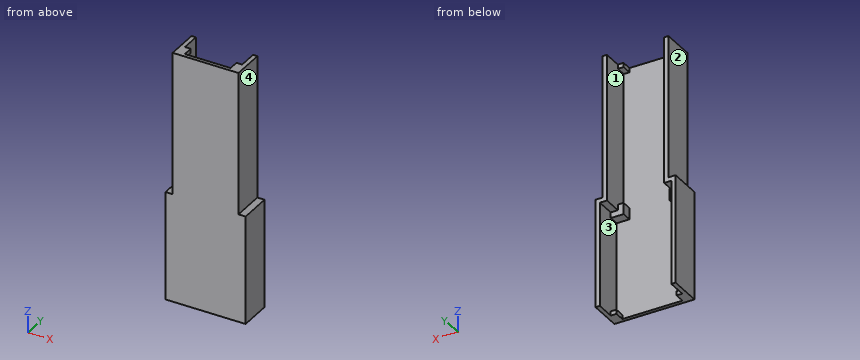
```python
from build123d import *

# Parameters (mm, degrees)
SKETCH1_W           = 46
SKETCH1_H           = 103
SKETCH1_W_2         = 56
SKETCH1_H_2         = 73
BOSS_EXTRUDE2_DEPTH = 2.5
BOSS_EXTRUDE3_DEPTH = 20
SKETCH4_W           = 3
SKETCH4_H           = 22.5
BOSS_EXTRUDE4_DEPTH = 5
SKETCH7_W           = 3
SKETCH7_H           = 22.5
BOSS_EXTRUDE5_DEPTH = 5
SKETCH8_W           = 4
SKETCH8_H           = 3
CUT_EXTRUDE1_DEPTH  = 13
SKETCH9_W           = 42
SKETCH9_H           = 3
CUT_EXTRUDE2_DEPTH  = 20
SKETCH10_W          = 32
SKETCH10_H          = 3
CUT_EXTRUDE3_DEPTH  = 20
SKETCH11_W          = 4
SKETCH11_H          = 4
BOSS_EXTRUDE6_DEPTH = 7


with BuildPart() as part:
    # Sketch1 → Boss-Extrude2 (new body)
    with BuildSketch(Plane(origin=(0, 0, 0), x_dir=(1, 0, 0), z_dir=(0, 1, 0))):
        with Locations((49.995495495, -98.63963964)):
            Rectangle(SKETCH1_W, SKETCH1_H)
        with Locations((49.995495495, -10.63963964)):
            Rectangle(SKETCH1_W_2, SKETCH1_H_2)
    extrude(amount=BOSS_EXTRUDE2_DEPTH)

    # Sketch3 → Boss-Extrude3 (add)
    with BuildSketch(Plane(origin=(0, 2.5, 0), x_dir=(1, 0, 0), z_dir=(0, 1, 0))):
        Polygon((24.995495495, -47.13963964), (24.995495495, 22.86036036), (74.995495495, 22.86036036), (74.995495495, -47.13963964), (77.995495495, -47.13963964), (77.995495495, 25.86036036), (21.995495495, 25.86036036), (21.995495495, -47.13963964), align=None)
        Polygon((29.995495495, -47.13963964), (26.995495495, -47.13963964), (26.995495495, -150.13963964), (72.995495495, -150.13963964), (72.995495495, -47.13963964), (69.995495495, -47.13963964), (69.995495495, -147.13963964), (29.995495495, -147.13963964), align=None)
    extrude(amount=BOSS_EXTRUDE3_DEPTH)

    # Sketch4 → Boss-Extrude4 (add)
    with BuildSketch(Plane.ZY.offset(-26.995495495)):
        with Locations((48.63963964, 11.25)):
            Rectangle(SKETCH4_W, SKETCH4_H)
    extrude(amount=BOSS_EXTRUDE4_DEPTH)

    # Sketch7 → Boss-Extrude5 (add)
    with BuildSketch(Plane(origin=(72.995495495, 0, 0), x_dir=(0, 0, -1), z_dir=(1, 0, 0))):
        with Locations((-48.63963964, 11.25)):
            Rectangle(SKETCH7_W, SKETCH7_H)
    extrude(amount=BOSS_EXTRUDE5_DEPTH)

    # Sketch8 → Cut-Extrude1 (cut)
    with BuildSketch(Plane(origin=(0, 22.5, 0), x_dir=(1, 0, 0), z_dir=(0, 1, 0))):
        with Locations((26.995495495, 24.36036036)):
            Rectangle(SKETCH8_W, SKETCH8_H)
        with Locations((72.995495495, 24.36036036)):
            Rectangle(SKETCH8_W, SKETCH8_H)
        with Locations((67.995495495, -148.63963964)):
            Rectangle(SKETCH8_W, SKETCH8_H)
        with Locations((31.995495495, -148.63963964)):
            Rectangle(SKETCH8_W, SKETCH8_H)
    extrude(amount=-CUT_EXTRUDE1_DEPTH, mode=Mode.SUBTRACT)

    # Sketch9 → Cut-Extrude2 (cut)
    with BuildSketch(Plane(origin=(0, 22.5, 0), x_dir=(1, 0, 0), z_dir=(0, 1, 0))):
        with Locations((49.995495495, 24.36036036)):
            Rectangle(SKETCH9_W, SKETCH9_H)
    extrude(amount=-CUT_EXTRUDE2_DEPTH, mode=Mode.SUBTRACT)

    # Sketch10 → Cut-Extrude3 (cut)
    with BuildSketch(Plane(origin=(0, 22.5, 0), x_dir=(1, 0, 0), z_dir=(0, 1, 0))):
        with Locations((49.995495495, -148.63963964)):
            Rectangle(SKETCH10_W, SKETCH10_H)
    extrude(amount=-CUT_EXTRUDE3_DEPTH, mode=Mode.SUBTRACT)

    # Sketch11 → Boss-Extrude6 (add)
    with BuildSketch(Plane(origin=(0, 2.5, 0), x_dir=(1, 0, 0), z_dir=(0, 1, 0))):
        with Locations((31.995495495, -49.13963964)):
            Rectangle(SKETCH11_W, SKETCH11_H)
        Polygon((24.995495495, -47.13963964), (29.995495495, -47.13963964), (33.995495495, -47.13963964), (33.995495495, -43.13963964), (24.995495495, -43.13963964), align=None)
        Polygon((65.995495495, -47.13963964), (69.995495495, -47.13963964), (74.995495495, -47.13963964), (74.995495495, -43.13963964), (65.995495495, -43.13963964), align=None)
        with Locations((67.995495495, -49.13963964)):
            Rectangle(SKETCH11_W, SKETCH11_H)
    extrude(amount=BOSS_EXTRUDE6_DEPTH)


solid = part.part
```
Read the model definition and answer for the solid it produces. Units are mm, in the model's axes. Face numbers are marked on the shaded views. Give positions to 0.01 mm unless a question says otherwise; leave off trailing zeros. Order: outer loops, then holes, each group sorted by start corner. A loop starts at its lowest first (then second) coordinate and runs counter-clockwise, first axis right, second up. Notation, with made-up numbers: (24.5, 26) -> (68.5, 26) arc R18 ccw to (68.5, 60) -> close; hole circle Ø8 at (72.25, 36). An arc over 180 degrees is marked (long way). One line per item, written item: value. Start each with the question number.
(1) The part is cut by section B-B (z = 112). Determine the outline of the cut face in (x, y).
(2) The part is cut by section A-A (y = 5.25). Determine the outline of the cut face in (x, z).
(3) Straight lines are drawn through the part: L1, parallel to X at y = 9.75, z = -8; L2, parallel to X at y = 12.5, z = 57.5; L3, parallel to Z at x = 28, y = 4.25. For each, find the intervals that lie inside material, in ascending order.
(4) Flat-ended cylindrical pins translate along their axes: P1, Ø1.5, axis at y = 6, z = 149, coming from the +X side; P2, Ø1.5, axis at x = 23.5, y = 15, coming from the +Z side; P3, Ø2.5, axis at x = 27, z = -23.5, coming from the +Y side. Find the tip coordinate at first contact, or state that the pin passes through.
(5) The part is cut by section C-C (y = 19.75). Determine the outline of the cut face in (x, z).
(6) The part is cut by section D-D (x = 45). Determine the outline of the cut face in (y, z).
(7) For a pull along X with two mould halves and no side action, classify the marked faces 1, 2, 3 and 4 as released by +X, released by -X, zero draft, split by the parting line, or undercut.
Taken from the geometry:
1. outline: (27, 0) -> (73, 0) -> (73, 22.5) -> (70, 22.5) -> (70, 2.5) -> (30, 2.5) -> (30, 22.5) -> (27, 22.5) -> close
2. outline: (22, -25.86) -> (29, -25.86) -> (29, -22.86) -> (25, -22.86) -> (25, 43.14) -> (34, 43.14) -> (34, 51.14) -> (30, 51.14) -> (30, 147.14) -> (34, 147.14) -> (34, 150.14) -> (27, 150.14) -> (27, 50.14) -> (22, 50.14) -> close; (66, 43.14) -> (75, 43.14) -> (75, -22.86) -> (71, -22.86) -> (71, -25.86) -> (78, -25.86) -> (78, 50.14) -> (73, 50.14) -> (73, 150.14) -> (66, 150.14) -> (66, 147.14) -> (70, 147.14) -> (70, 51.14) -> (66, 51.14) -> close
3. L1: 22 to 25, 75 to 78
3. L2: 27 to 30, 70 to 73
3. L3: -25.86 to -22.86, 43.14 to 150.14
4. P1: x = 73
4. P2: z = 50.14
4. P3: y = 9.5
5. outline: (22, -25.86) -> (25, -25.86) -> (25, 47.14) -> (30, 47.14) -> (30, 150.14) -> (27, 150.14) -> (27, 50.14) -> (22, 50.14) -> close; (70, 47.14) -> (75, 47.14) -> (75, -25.86) -> (78, -25.86) -> (78, 50.14) -> (73, 50.14) -> (73, 150.14) -> (70, 150.14) -> close
6. outline: (0, -25.86) -> (2.5, -25.86) -> (2.5, 150.14) -> (0, 150.14) -> close
7. face 1: undercut
7. face 2: released by -X
7. face 3: undercut
7. face 4: released by +X
